from build123d import *

# Parameters (mm, degrees)
SKETCH1_R           = 9
SKETCH1_R_2         = 3
BOSS_EXTRUDE1_DEPTH = 1
SKETCH1_3_R         = 3
SKETCH1_3_R_2       = 2
BOSS_EXTRUDE2_DEPTH = 4
SKETCH1_4_R         = 2
BOSS_EXTRUDE3_DEPTH = 2
SKETCH2_R           = 0.75
CUT_EXTRUDE1_DEPTH  = 2
SKETCH3_R           = 0.75
CUT_EXTRUDE2_DEPTH  = 14.076696831


with BuildPart() as part:
    # Sketch1 → Boss-Extrude1 (new body)
    with BuildSketch(Plane.XY):
        Circle(SKETCH1_R)
        Circle(SKETCH1_R_2, mode=Mode.SUBTRACT)
    extrude(amount=BOSS_EXTRUDE1_DEPTH)

    # Sketch1_3 → Boss-Extrude2 (add)
    with BuildSketch(Plane.XY):
        Circle(SKETCH1_3_R)
        Circle(SKETCH1_3_R_2, mode=Mode.SUBTRACT)
    extrude(amount=BOSS_EXTRUDE2_DEPTH)

    # Sketch1_4 → Boss-Extrude3 (add)
    with BuildSketch(Plane.XY):
        Circle(SKETCH1_4_R)
    extrude(amount=BOSS_EXTRUDE3_DEPTH)

    # Sketch2 → Cut-Extrude1 (cut)
    with BuildSketch(Plane.XY.offset(2)):
        Circle(SKETCH2_R)
    extrude(amount=-CUT_EXTRUDE1_DEPTH, mode=Mode.SUBTRACT)

    # Sketch3 → Cut-Extrude2 (cut, through all)
    with BuildSketch(Plane.XY.offset(1)):
        with Locations((3.75, 0)):
            Circle(SKETCH3_R)
        with Locations((5.75, 0)):
            Circle(SKETCH3_R)
        with Locations((7.75, 0)):
            Circle(SKETCH3_R)
        with Locations(Location((-3.75, 0, 0), (0, 0, 0.000836859))):
            Circle(SKETCH3_R)
        with Locations(Location((-5.75, 0, 0), (0, 0, 180))):
            Circle(SKETCH3_R)
        with Locations(Location((-7.75, 0, 0), (0, 0, 180))):
            Circle(SKETCH3_R)
        with Locations((0, 3.75)):
            Circle(SKETCH3_R)
        with Locations((0, 5.75)):
            Circle(SKETCH3_R)
        with Locations((0, 7.75)):
            Circle(SKETCH3_R)
        with Locations(Location((0, -3.75, 0), (0, 0, 90.000836859))):
            Circle(SKETCH3_R)
        with Locations(Location((0, -5.75, 0), (0, 0, 180))):
            Circle(SKETCH3_R)
        with Locations(Location((0, -7.75, 0), (0, 0, 180))):
            Circle(SKETCH3_R)
    extrude(amount=-CUT_EXTRUDE2_DEPTH, mode=Mode.SUBTRACT)


solid = part.part
The listing builds one solid part. Answer for the finished solid, in the listing's coordinates (mm). A direction names the side the tool comes from. Round coordinates to 2 decimals unless told otherwise and drop trailing zeros. Order: outer loops, then holes, each group sorted by start corner. A loop starts at its lowest first (then second) coordinate and runs counter-clockwise, first axis right, second up. Notation, with made-up numbers: (58.5, 59) -> (101.5, 59) arc R19 ccw to (101.5, 84) -> close; hole circle Ø10 at (2, 43). An arc over 180 degrees is marked (long way). Write each question's results on one line, items separated by ' | '. Start each with the question number.
Q1. Find section A-A (x = -3.75). Determine the outline of the cut face in (y, z), then the cut area to 3 significant figures.
Q2. The mould has two halves that part along X. Classify faces 3 (the cylindrical face through (-1.172, 8.923, 0.493)), 4 (the flat face through (1, -2, 4)), 5 (the cylindrical face through (-0.55, 8.26, 0.51)): pulls with the +X half, pulls with the -X half, needs draft (parallel to the pull), parting line crosses it, or undercut.
Q3. Straight lines are drawn through the part: probe 1 along Y at (x, z) = (0, 3.2); probe 2 along Y at (x, z) = (-7.75, 0.55); probe 3 along Z at (x, y) = (1.75, 4.75). For each, find the intervals that lie inside material, in ascending order. Write a range as from..to.
Q4. Find section B-B (y = 7.75). Determine the outline of the cut face in (x, z), then the cut area to 3 significant figures.
Q5. Which of the six approach directions +Z, -Z, +X, -X, +Y, -Y give full straight-line access (tool end or side, diameter ignored) to faces 1 (the cylindrical face through (-7, 0, 0.5)), 2 (the flat face through (4, -2, 1))?
Q6. Find section C-C (z = 3). Determine the outline of the cut face in (x, y).
Q7. Find section D-D (z = 0.3). Give the number of separate pieces and of enclosed holes in the cut face, then the cut area to 3 significant figures.
Q8. Each of these flat-tipped pins is pushed along its axis until it touches: pin 1 (2 mm diameter, centred on y = 1, z = 2.5, fed in from -X); pin 2 (2 mm diameter, centred on x = -4, y = 1.5, fed in from +Z); pin 3 (3 mm diameter, centred on x = 0, y = 0, fed in from +Z). Where does it stop, or does it pass through?
Worked answers:
1) outline: (-8.18, 0) -> (-0.75, 0) -> (-0.75, 1) -> (-8.18, 1) -> close; (0.75, 0) -> (8.18, 0) -> (8.18, 1) -> (0.75, 1) -> close | area: 14.9 mm2
2) face 3: parting line crosses it | face 4: needs draft | face 5: undercut
3) probe 1: y = -3..-2, 2..3 | probe 2: y = -4.58..-0.75, 0.75..4.58 | probe 3: z = 0..1
4) outline: (-4.58, 0) -> (-0.75, 0) -> (-0.75, 1) -> (-4.58, 1) -> close; (0.75, 0) -> (4.58, 0) -> (4.58, 1) -> (0.75, 1) -> close | area: 7.65 mm2
5) face 1: +Z, -Z | face 2: +Z
6) outline: circle Ø6 at (0, 0); hole circle Ø4 at (0, 0)
7) separate pieces: 1 | enclosed holes: 13 | area: 231 mm2
8) pin 1: stops at x = -3 | pin 2: stops at z = 1 | pin 3: stops at z = 2
